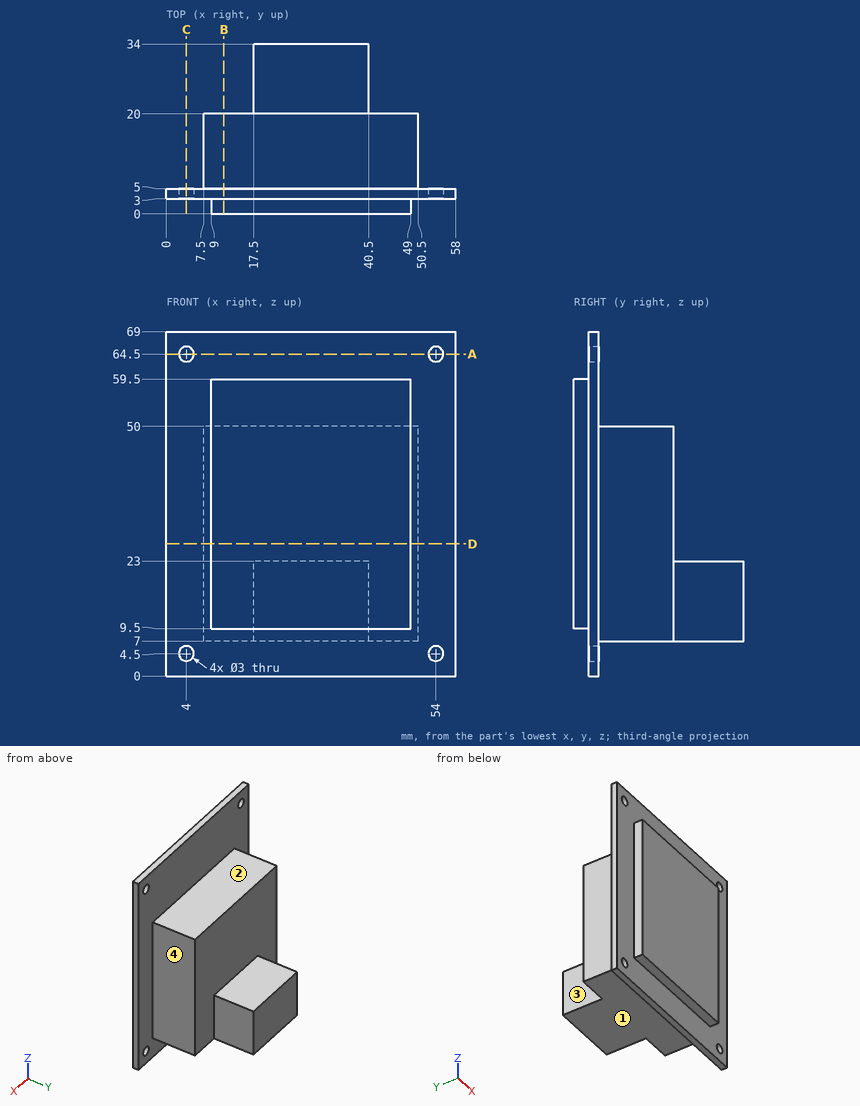
Input: dimensioned drawing with shaded views. Units: mm. Origin: part minimum x, y, z. A direction names the side the tool comes from. Coordinates: 2 decimals unless noted, no trailing zeros. Order: outer loops, then holes, each group sorted by start corner. A loop starts at its lowest first (then second) coordinate and runs counter-clockwise, first axis right, second up. Notation, with made-up numbers: (45, 3) - (99, 3) arc R23 cw to (99, 36) - close; hole circle Ø6 at (81.5, 1). An arc over 180 degrees is marked (long way). Return JSON: item names as keys, results as strings. Group by question number.
1. Cut plane D-D (z = 26.5). Output: boundary loops of the cut face in (x, y), plus the area to 3 significant figures.
2. Material intervals for line 1 along X through (y, z) = (3.75, 4.5); line 2 along Y through (x, z) = (31, 60); line 3 along Y through (x, z) = (8.5, 31), sorted ascending. Write a range as [from, to].
3. Cut plane B-B (x = 11.5). Output: boundary loops of the cut face in (y, z), plus the area to 3 significant figures.
4. Cut plane A-A (z = 64.5). Output: boundary loops of the cut face in (x, y), plus the area to 3 significant figures.
5. Set-up query: the marked faces 1, 2, 3 and 4. Return all of +Z, -Z, +X, -X, +Y, -Y with unobstructed straight access to the full face (end or side cutting, diameter ignored); none if empty.
6. Pin query (flat end, axial travel): pin 1 (0.9 mm diameter, centred on y = 1, z = 30.5, fed in from -X); pin 2 (14.5 mm diameter, centred on x = 27, y = 22, fed in from -Z); pin 3 (5 mm diameter, centred on x = 4, z = 4.5, fed in from +Y); pin 4 (2.5 mm diameter, centred on x = 4, z = 64.5, fed in from +Y). Return the tip coordinate at first contact, or that it passes through.
7. Cut plane C-C (x = 4). Output: boundary loops of the cut face in (y, z).
Resolved:
{
 "1": {"outline": "(0, 3) - (9, 3) - (9, 0) - (49, 0) - (49, 3) - (58, 3) - (58, 5) - (50.5, 5) - (50.5, 20) - (7.5, 20) - (7.5, 5) - (0, 5) - close", "area": "881 mm²"},
 "2": {"line 1": "x = [0, 2.5], [5.5, 52.5], [55.5, 58]", "line 2": "y = [3, 5]", "line 3": "y = [3, 20]"},
 "3": {"outline": "(0, 9.5) - (3, 9.5) - (3, 0) - (5, 0) - (5, 7) - (20, 7) - (20, 50) - (5, 50) - (5, 69) - (3, 69) - (3, 59.5) - (0, 59.5) - close", "area": "933 mm²"},
 "4": {"outline": "(0, 3) - (2.5, 3) - (2.5, 5) - (0, 5) - close; (5.5, 3) - (52.5, 3) - (52.5, 5) - (5.5, 5) - close; (55.5, 3) - (58, 3) - (58, 5) - (55.5, 5) - close", "area": "104 mm²"},
 "5": {"face 1": "-Z, +X, -X, +Y", "face 2": "+Z, +X, -X, +Y", "face 3": "+Z, -Z, -X, +Y", "face 4": "+Z, -Z, +X, +Y"},
 "6": {"pin 1": "stops at x = 9", "pin 2": "stops at z = 7", "pin 3": "stops at y = 5", "pin 4": "passes through"},
 "7": {"outline": "(3, 0) - (5, 0) - (5, 3) - (3, 3) - close; (3, 6) - (5, 6) - (5, 63) - (3, 63) - close; (3, 66) - (5, 66) - (5, 69) - (3, 69) - close"}
}
